from build123d import *

# Parameters (mm, degrees)
EXTRUDE_1_OUTLINE_R = 0.19875
EXTRUDE_1_DEPTH     = 0.3975
SCALE_3_SCALE       = 25
SKETCH_2_W          = 6
SKETCH_2_H          = 7.65
CUT_EXTRUDE_1_DEPTH = 10


# Read off the part's stored shape, not the designer's step: 凸台-拉伸1
with BuildPart() as part:
    # 凸台-拉伸1 outline → 凸台-拉伸1 (new body)
    with BuildSketch(Plane.XY):
        with BuildLine():
            Line((0.281074946, 0.562149891), (2.103665998, 2.384740944))
            ThreePointArc((2.103665998, 2.384740944), (2.027732849, 2.449632522), (1.949799165, 2.512107326))
            ThreePointArc((1.949799165, 2.512107326), (0, 1.714699128), (-1.949799165, 2.512107326))
            ThreePointArc((-1.949799165, 2.512107326), (-2.027732849, 2.449632522), (-2.103665998, 2.384740944))
            Line((-2.103665998, 2.384740944), (-0.281074946, 0.562149891))
            ThreePointArc((-0.281074946, 0.562149891), (-0.281074946, 0.281074946), (-0.562149891, 0.281074946))
            Line((-0.562149891, 0.281074946), (-2.384740944, 2.103665998))
            ThreePointArc((-2.384740944, 2.103665998), (-2.449632522, 2.027732849), (-2.512107326, 1.949799165))
            ThreePointArc((-2.512107326, 1.949799165), (-1.714699128, 0), (-2.512107326, -1.949799165))
            ThreePointArc((-2.512107326, -1.949799165), (-2.449632522, -2.027732849), (-2.384740944, -2.103665998))
            Line((-2.384740944, -2.103665998), (-0.562149891, -0.281074946))
            ThreePointArc((-0.562149891, -0.281074946), (-0.281074946, -0.281074946), (-0.281074946, -0.562149891))
            Line((-0.281074946, -0.562149891), (-2.103665998, -2.384740944))
            ThreePointArc((-2.103665998, -2.384740944), (-2.027732849, -2.449632522), (-1.949799165, -2.512107326))
            ThreePointArc((-1.949799165, -2.512107326), (0, -1.714699128), (1.949799165, -2.512107326))
            ThreePointArc((1.949799165, -2.512107326), (2.027732849, -2.449632522), (2.103665998, -2.384740944))
            Line((2.103665998, -2.384740944), (0.281074946, -0.562149891))
            ThreePointArc((0.281074946, -0.562149891), (0.281074946, -0.281074946), (0.562149891, -0.281074946))
            Line((0.562149891, -0.281074946), (2.384740944, -2.103665998))
            ThreePointArc((2.384740944, -2.103665998), (2.449632522, -2.027732849), (2.512107326, -1.949799165))
            ThreePointArc((2.512107326, -1.949799165), (1.714699128, 0), (2.512107326, 1.949799165))
            ThreePointArc((2.512107326, 1.949799165), (2.449632522, 2.027732849), (2.384740944, 2.103665998))
            Line((2.384740944, 2.103665998), (0.562149891, 0.281074946))
            ThreePointArc((0.562149891, 0.281074946), (0.281074946, 0.281074946), (0.281074946, 0.562149891))
        make_face()
        Circle(EXTRUDE_1_OUTLINE_R, mode=Mode.SUBTRACT)
    extrude(amount=EXTRUDE_1_DEPTH)


with BuildPart() as part_1:
    # 缩放比例3: scaled about (0, 0, 0.19875)
    add(part.part.scale(SCALE_3_SCALE).moved(Location((0, 0, -4.77))))

    # 草图2 → 切除-拉伸1 (cut)
    with BuildSketch(Plane.XY.offset(5.1675)):
        with Locations((0, 3.825)):
            Rectangle(SKETCH_2_W, SKETCH_2_H)
    extrude(amount=-CUT_EXTRUDE_1_DEPTH, mode=Mode.SUBTRACT)


solid = part_1.part
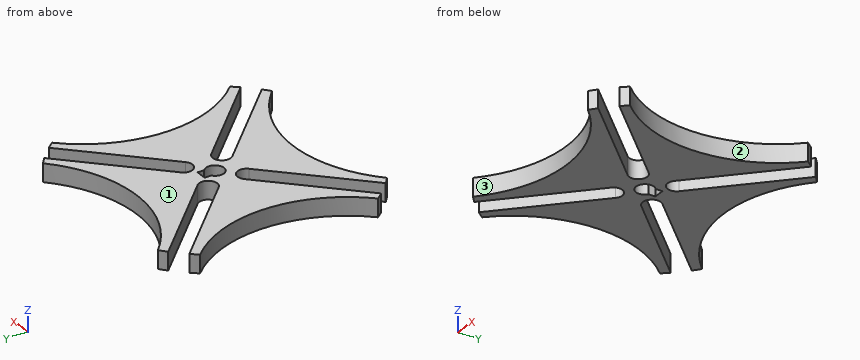
Can you work these out from the model? Positions are in its coordinate system, mm. Face numbers are marked on the shaded views. Round coordinates to 2 decimals unless told otherwise and drop trailing zeros. Order: outer loops, then holes, each group sorted by start corner. A loop starts at its lowest first (then second) coordinate and runs counter-clockwise, first axis right, second up. Notation, with made-up numbers: (-14.75, -20.5) - (17.25, -20.5) arc R28 cw to (17.25, -2.5) - close; hole circle Ø4 at (51.25, 58). An arc over 180 degrees is marked (long way). Answer in a Markdown table with one row per item.
(1) If we mould it in two halves opening along X, with no side actions, what happens to the marked faces 1, 2 and 3? For each: released by +X, released by -X, zero draft, split by the parting line, or undercut.
From the geometry:
| item | result |
|---|---|
| face 1 | zero draft |
| face 2 | released by +X |
| face 3 | undercut |
(2) Please list where these lines run through material, in increasing order: L1, parallel to X at y = 33.5, z = 1.5; L2, parallel to Y at x = 31, z = 0.5; L3, parallel to X at y = 27, z = -1.25. Write a range as from..to.
From the geometry:
| item | result |
|---|---|
| L1 | x = -51.47..-40.53, -26.47..26.47, 40.53..51.47 |
| L2 | y = -50.16..-38.03, -23.97..23.97, 38.03..50.16 |
| L3 | x = -48.32..-34.03, -19.97..19.97, 34.03..48.32 |
(3) For P1, Ø16, axis at x = 0, y = 0, coming from the +Z side; P2, Ø2, axis at x = -46, z = -0.5, coming from the -Y side; P3, Ø3, axis at y = 6, z = -1, coming from the -X side; P4, Ø1.8, axis at x = -1, z = 0, coming from the -Y side, each with a flat end and sliding along its axis, tell me the tip position at first contact or that it passes through.
From the geometry:
| item | result |
|---|---|
| P1 | stops at z = 5.17 |
| P2 | stops at y = -61.15 |
| P3 | stops at x = -43.27 |
| P4 | stops at y = -42.89 |
(4) Suppose I cut it at A-A, the plane y = 0. Please give me the cut outline in (x, z).
From the geometry:
| item | result |
|---|---|
| outline | (-42.87, -4.77) - (-4.97, -4.77) - (-4.97, 5.17) - (-42.87, 5.17) - close; (4.97, -4.77) - (42.87, -4.77) - (42.87, 5.17) - (4.97, 5.17) - close |
(5) Suppose I cut it at B-B, the plane x = 0. Please give me the cut outline in (y, z).
From the geometry:
| item | result |
|---|---|
| outline | (-42.87, -4.77) - (-4.97, -4.77) - (-4.97, 5.17) - (-42.87, 5.17) - close; (7.65, -4.77) - (42.87, -4.77) - (42.87, 5.17) - (7.65, 5.17) - close |
(6) Suppose I cut it at D-D, the plane y = -33. Please give me the cut outline in (x, z), plus the area to 3 significant figures.
From the geometry:
| item | result |
|---|---|
| outline | (-51.19, -4.77) - (-40.03, -4.77) - (-40.03, 5.17) - (-51.19, 5.17) - close; (-25.97, -4.77) - (25.97, -4.77) - (25.97, 5.17) - (-25.97, 5.17) - close; (40.03, -4.77) - (51.19, -4.77) - (51.19, 5.17) - (40.03, 5.17) - close |
| area | 738 mm2 |
